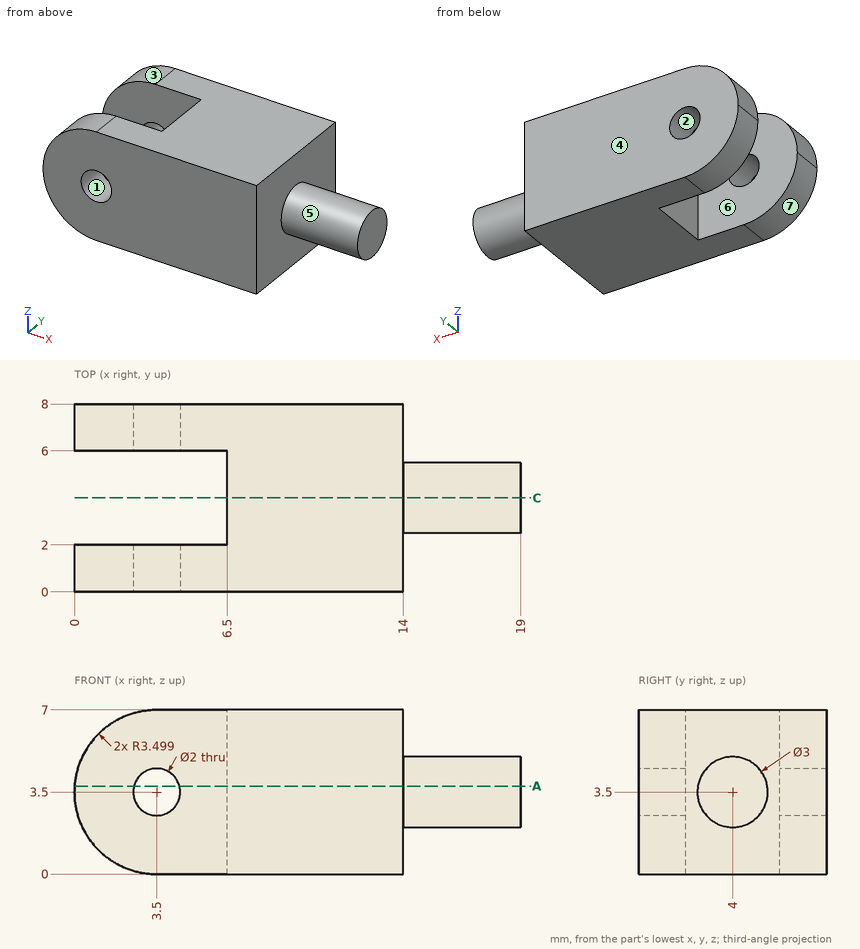
Input: dimensioned drawing with shaded views. Units: mm. Origin: part minimum x, y, z. A direction names the side the tool comes from. Coordinates: 2 decimals unless noted, no trailing zeros. Order: outer loops, then holes, each group sorted by start corner. A loop starts at its lowest first (then second) coordinate and runs counter-clockwise, first axis right, second up.
Item 1: Section query A-A (z = 3.75). Output: boundary loops of the cut face in (x, y).
Answer:
outline: (0.01, 0) - (2.53, 0) - (2.53, 2) - (0.01, 2) - close; (0.01, 6) - (2.53, 6) - (2.53, 8) - (0.01, 8) - close; (4.47, 0) - (14, 0) - (14, 2.52) - (19, 2.52) - (19, 5.48) - (14, 5.48) - (14, 8) - (4.47, 8) - (4.47, 6) - (6.5, 6) - (6.5, 2) - (4.47, 2) - close
Item 2: Access query for the marked faces 5, 6 and 7. Directions: +Z, -Z, +X, -X, +Y, -Y. A direction counts if a zero-diameter tool reaches every point of the face in a straight line with its end or side. Return the directions, or none.
Answer:
face 5: +X
face 6: +Z, -Z, -X
face 7: -Z, -X, +Y, -Y
Item 3: Material intervals for line 1 along Y through (x, z) = (6.25, 6); line 2 along X through (y, z) = (7.1, 3.5); line 3 along Z through (x, y) = (3.5, 7.65), sorted ascending.
Answer:
line 1: y = 0 to 2, 6 to 8
line 2: x = 0 to 2.5, 4.5 to 14
line 3: z = 0 to 2.5, 4.5 to 7
Item 4: Contact query for flat-ended pins moving along their axis: P1, Ø1.6, axis at x = 3.5, z = 3.5, coming from the +Y side; P2, Ø1, axis at y = 4, z = 3.5, coming from the -X side. Output: stop coordinate, or through.
Answer:
P1: passes through
P2: stops at x = 6.5
Item 5: Draft query along Z for the marked faces 1, 2, 3 and 4. Return one class per face: released by +Z, released by -Z, zero draft, split by the parting line, or undercut.
Answer:
face 1: undercut
face 2: undercut
face 3: released by +Z
face 4: zero draft
Item 6: Section query C-C (y = 4). Output: boundary loops of the cut face in (x, z).
Answer:
outline: (6.5, 0) - (14, 0) - (14, 2) - (19, 2) - (19, 5) - (14, 5) - (14, 7) - (6.5, 7) - close
